Read the model definition and answer for the solid it produces. Units are mm, in the model's axes. Face numbers are marked on the shaded views. A direction names the side the tool comes from. Coordinates: 2 decimals unless noted, no trailing zeros. Write each loop counter-clockwise with the first axis right and the second up, starting at its lowest first coordinate (ties: lowest second). Pieces come first, ordered by that corner, then holes. Notation, with made-up numbers: (81, 2.25) - (135, 2.25) arc R33 ccw to (135, 41.25) - close; hole circle Ø4 at (42.25, 56.25). An arc over 180 degrees is marked (long way). Use a Markdown table: item, result.
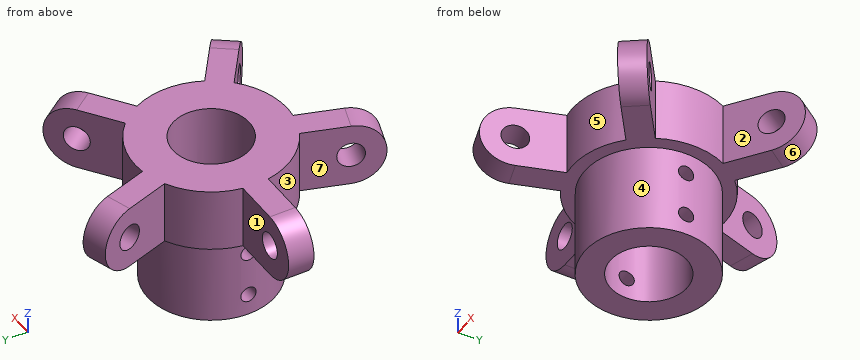
from build123d import *

# Parameters (mm, degrees)
F3_DEPTH      = 1
F4_R          = 1
F5_DEPTH      = 7.001
F6_COUNT      = 5
F7_R          = 0.6
F8_DEPTH      = 12.001
F8_DEPTH_BACK = 10.2969891848


with BuildPart() as f1:
    # F0 (on Front) → F1 (revolve)
    with BuildSketch(Plane.XZ):
        Polygon((-3, -7), (-3, 5), (-6, 5), (-6, 0), (-5, 0), (-5, -7), align=None)
    revolve(axis=Axis((0, 0, -4.9457359128), (0, 0, -1)))

    # F2 (on Front) → F3 (join, symmetric)
    with BuildSketch(Plane.XZ):
        with BuildLine():
            ThreePointArc((-7, 2.5), (-7.732233047, 4.267766953), (-9.5, 5))
            ThreePointArc((-9.5, 5), (-12, 2.5), (-9.5, 0))
            ThreePointArc((-9.5, 0), (-7.732233047, 0.732233047), (-7, 2.5))
        make_face()
        with BuildLine():
            Line((-5, 5), (-9.5, 5))
            ThreePointArc((-9.5, 5), (-7.732233047, 4.267766953), (-7, 2.5))
            ThreePointArc((-7, 2.5), (-7.732233047, 0.732233047), (-9.5, 0))
            Line((-9.5, 0), (-5, 0))
            Line((-5, 0), (-5, 5))
        make_face()
    extrude(amount=F3_DEPTH, both=True)

    # F4 (on face) → F5 (cut, through all)
    with BuildSketch(Plane.XZ.offset(1)):
        with Locations((-9.5, 2.5)):
            Circle(F4_R)
    extrude(amount=-F5_DEPTH, mode=Mode.SUBTRACT)

    # F6: F1 ×5 about axis
    f6_axis = Axis((0, 0, -7), (0, 0, 1))


with BuildPart() as f1_1:
    add(f1.part)
    for i in range(1, F6_COUNT):
        add(f1.part.rotate(f6_axis, i * 360 / F6_COUNT))

    # F7 (on Right) → F8 (cut, two sides)
    with BuildSketch(Plane.YZ) as f8_sk:
        with Locations((0, -1.7)):
            Circle(F7_R)
        with Locations((0, -5.3)):
            Circle(F7_R)
    extrude(amount=-F8_DEPTH, mode=Mode.SUBTRACT)
    extrude(f8_sk.sketch, amount=F8_DEPTH_BACK, mode=Mode.SUBTRACT)


solid = f1_1.part
(1) Each of these flat-tipped pins is pushed along its axis until it touches: P1, Ø5, axis at y = 3, z = 3.5, coming from the +X side; P2, Ø1, axis at y = -5.5, z = 2, coming from the -X side; P3, Ø4, axis at x = -8, z = 2, coming from the +Y side. Where does it stop, or does it pass through?
Report:
| item | result |
|---|---|
| P1 | stops at x = 9.27 |
| P2 | stops at x = -3.32 |
| P3 | stops at y = 1 |
(2) A cutting plane is placed at B-B, the plane x = 0. Write down the section's boundary in (y, z), and give its area (3 significant figures).
Report:
| item | result |
|---|---|
| outline | (-6, 0) - (-5, 0) - (-5, -7) - (-3, -7) - (-3, 5) - (-6, 5) - close; (3, -7) - (5, -7) - (5, 0) - (6, 0) - (6, 5) - (3, 5) - close |
| area | 58.0 mm² |
(3) A cutting plane is placed at C-C, the plane z = -5.3. Write down the section's boundary in (x, y), and give its area (3 significant figures).
Report:
| item | result |
|---|---|
| outline | (-4.96, -0.6) arc R5 ccw to (4.96, -0.6) - (2.94, -0.6) arc R3 cw to (-2.94, -0.6) - close; (-4.96, 0.6) - (-2.94, 0.6) arc R3 cw to (2.94, 0.6) - (4.96, 0.6) arc R5 ccw to start |
| area | 45.4 mm² |
(4) A cutting plane is placed at D-D, the plane z = -3. Write down the section's boundary in (x, y), and give its area (3 significant figures).
Report:
| item | result |
|---|---|
| outline | circle Ø10 at (0, 0); hole circle Ø6 at (0, 0) |
| area | 50.3 mm² |
(5) The mould has two halves that part along Y. Classify the marked faces 5, 6 and 7: pulls with the +Y half, pulls with the -Y half, needs draft (parallel to the pull), parting line crosses it, or undercut.
Report:
| item | result |
|---|---|
| face 5 | pulls with the -Y half |
| face 6 | pulls with the +Y half |
| face 7 | undercut |
(6) Straight lines are drawn through the part: L1, parallel to Z at x = 3.6, y = 0; L2, parallel to Y at x = 0, z = 2.5; L3, parallel to Z at x = -2.75, y = 9. For each, find the intervals that lie inside material, in ascending order.
Report:
| item | result |
|---|---|
| L1 | z = -7 to -5.9, -4.7 to -2.3, -1.1 to 5 |
| L2 | y = -6 to -3, 3 to 6 |
| L3 | z = 0 to 1.5, 3.5 to 5 |
(7) A cutting plane is placed at A-A, the plane y = 0. Count the separate pieces of the cut face and the enclosed holes in it, and give its area (3 significant figures).
Report:
| item | result |
|---|---|
| separate pieces | 6 |
| enclosed holes | 1 |
| area | 72.6 mm² |
(8) For the marked faces 1, 2, 3 and 4, determine the directions among +Z, -Z, +X, -X, +Y, -Y from which every point of the face is accessible in a straight line to the end or side of a thin tool.
Report:
| item | result |
|---|---|
| face 1 | +Z, -Z, -X, +Y |
| face 2 | +Z, -Z, +X |
| face 3 | +Z, -Z, -X |
| face 4 | -Z |
